```python
from build123d import *

# Parameters (mm, degrees)
SKETCH1_R           = 0.5
SKETCH1_R_2         = 0.75
BOSS_EXTRUDE1_DEPTH = 1.6
BOSS_EXTRUDE2_START = 2.5
SKETCH2_R           = 3.25
BOSS_EXTRUDE2_DEPTH = 2.5
SKETCH4_R           = 1
CUT_EXTRUDE1_DEPTH  = 17.359171739
CUT_EXTRUDE2_DEPTH  = 3
SKETCH3_R           = 2.5
CUT_EXTRUDE3_DEPTH  = 0.75


with BuildPart() as part:
    # Sketch1 → Boss-Extrude1 (new body)
    with BuildSketch(Plane(origin=(0, 0, 0), x_dir=(1, 0, 0), z_dir=(0, 1, 0))):
        with BuildLine():
            Line((2.218529919, 2.375), (13.5, 2))
            ThreePointArc((13.5, 2), (15.499725592, 0.033129364), (13.566249638, -1.998902445))
            Line((13.566249638, -1.998902445), (2.218529919, -2.375))
            ThreePointArc((2.218529919, -2.375), (-3.25, 0), (2.218529919, 2.375))
        make_face()
        with Locations(Location((13.5, 0, 0), (0, 0, 270))):
            Circle(SKETCH1_R, mode=Mode.SUBTRACT)
        with Locations(Location((11.5, 0, 0), (0, 0, 270))):
            Circle(SKETCH1_R, mode=Mode.SUBTRACT)
        with Locations(Location((9.5, 0, 0), (0, 0, 270))):
            Circle(SKETCH1_R_2, mode=Mode.SUBTRACT)
        with Locations(Location((7.5, 0, 0), (0, 0, 270))):
            Circle(SKETCH1_R, mode=Mode.SUBTRACT)
        with Locations(Location((5.5, 0, 0), (0, 0, 270))):
            Circle(SKETCH1_R, mode=Mode.SUBTRACT)
    extrude(amount=BOSS_EXTRUDE1_DEPTH)

    # Sketch2 → Boss-Extrude2 (add)
    with BuildSketch(Plane.XZ.offset(BOSS_EXTRUDE2_START)):
        with Locations(Location((0, 0, 0), (0, 0, 270))):
            Circle(SKETCH2_R)
    extrude(amount=-BOSS_EXTRUDE2_DEPTH)

    # Sketch4 → Cut-Extrude1 (cut, through all)
    with BuildSketch(Plane(origin=(0, 1.6, 0), x_dir=(1, 0, 0), z_dir=(0, 1, 0))):
        with Locations(Location((0, 0, 0), (0, 0, 270))):
            Circle(SKETCH4_R)
    extrude(amount=-CUT_EXTRUDE1_DEPTH, mode=Mode.SUBTRACT)

    # Sketch5 → Cut-Extrude2 (cut)
    with BuildSketch(Plane.XZ.offset(2.5)):
        Polygon((0, 2), (0.374241043, 1.760665681), (0.813473286, 1.827090915), (1.058013454, 1.45623059), (1.486289651, 1.338261213), (1.558845727, 0.9), (1.902113033, 0.618033989), (1.790139412, 0.188151234), (1.989043791, -0.209056927), (1.711901729, -0.55623059), (1.732050808, -1), (1.337660686, -1.204435091), (1.175570505, -1.618033989), (0.732125958, -1.644381824), (0.415823382, -1.956295201), (0, -1.8), (-0.415823382, -1.956295201), (-0.732125958, -1.644381824), (-1.175570505, -1.618033989), (-1.337660686, -1.204435091), (-1.732050808, -1), (-1.711901729, -0.55623059), (-1.989043791, -0.209056927), (-1.790139412, 0.188151234), (-1.902113033, 0.618033989), (-1.558845727, 0.9), (-1.486289651, 1.338261213), (-1.058013454, 1.45623059), (-0.813473286, 1.827090915), (-0.374241043, 1.760665681), align=None)
    extrude(amount=-CUT_EXTRUDE2_DEPTH, mode=Mode.SUBTRACT)

    # Sketch3 → Cut-Extrude3 (cut)
    with BuildSketch(Plane(origin=(0, 1.6, 0), x_dir=(1, 0, 0), z_dir=(0, 1, 0))):
        with Locations(Location((0, 0, 0), (0, 0, 270))):
            Circle(SKETCH3_R)
    extrude(amount=-CUT_EXTRUDE3_DEPTH, mode=Mode.SUBTRACT)


solid = part.part
```
The listing builds one solid part. Answer for the finished solid, in the listing's coordinates (mm). A direction names the side the tool comes from. Coordinates: 2 decimals unless noted, no trailing zeros. Loops run counter-clockwise (first coordinate to the right, second up) from the corner with the lowest first, then second, coordinate; pieces in that order, holes last. Notation, with made-up numbers: M 72.5,60.5 L 103.5,60.5 A19 ccw 103.5,83.5 Z; hole C 44,55.5 d1. An arc over 180 degrees is marked long. Answer as a JSON object with one key per item and string values. Group by question number.
Item 1: Which of the six approach directions +Z, -Z, +X, -X, +Y, -Y give full straight-line access (tool end or side, diameter ignored) to faces 5 (the face through (-1, 0.85, 1)), 6 (the face through (6.3, 1.6, 0))?
Item 2: Section B-B (x = 5.5) is taken. Write down the section's boundary in (y, z).
Item 3: Section D-D (x = 9.75) is taken. Write down the section's boundary in (y, z).
Item 4: Consider L1, parallel to Y at x = 5.25, z = -1; L2, parallel to X at y = -2.05, z = 1; L3, parallel to X at y = 1.1, z = 1.75. Determine where each line is inside the solid, lowest interval first.
Item 5: Each of these flat-tipped pins is pushed along its axis until it touches: P1, Ø1, axis at y = -1, z = 2, coming from the -X side; P2, Ø1.5, axis at y = -1.5, z = 0, coming from the +X side; P3, Ø2.5, axis at x = 0, z = 0, coming from the +Y side. Where does it stop, or does it pass through?
Item 6: Determine the mould class of faces 1 (the face through (0, -2.5, -2)), 2 (the face through (15.5, 0.79, -0.08)), 3 (the face through (-1, 0.5, -1)), 4 (the face through (-2.44, 1.23, -0.54)) for opening direction X: +X half, -X half, draft (parallel to the pull), parting line (faces both ways), or undercut.
Item 7: Section A-A (y = 1.2) is taken. Write down the section's boundary in (x, z) (3 decimals).
Solved:
{
 "1": {"face 5": "+Y", "face 6": "+Z, -Z, +X, -X, +Y"},
 "2": {"outline": "M 0,-2.27 L 1.6,-2.27 L 1.6,-0.5 L 0,-0.5 Z; M 0,0.5 L 1.6,0.5 L 1.6,2.27 L 0,2.27 Z"},
 "3": {"outline": "M 0,-2.12 L 1.6,-2.12 L 1.6,-0.71 L 0,-0.71 Z; M 0,0.71 L 1.6,0.71 L 1.6,2.13 L 0,2.13 Z"},
 "4": {"L1": "y = 0 to 1.6", "L2": "x = -3.09 to -1.54, 1.54 to 3.09", "L3": "x = -2.74 to -1.79, 1.79 to 14.47"},
 "5": {"P1": "stops at x = -2.88", "P2": "stops at x = 3.25", "P3": "stops at y = 0.85"},
 "6": {"face 1": "draft", "face 2": "+X half", "face 3": "undercut", "face 4": "undercut"},
 "7": {"outline": "M 2.219,-2.375 L 13.5,-2 A2 ccw 13.566,1.999 L 2.219,2.375 A3.25 ccw long Z; hole C 0,0 d5; hole C 5.5,0 d1; hole C 7.5,0 d1; hole C 9.5,0 d1.5; hole C 11.5,0 d1; hole C 13.5,0 d1"}
}
